For this review, take the finished solid that the model builds, in its own axes (mm). Face numbers are marked on the shaded views. A direction names the side the tool comes from. Round coordinates to 2 decimals unless told otherwise and drop trailing zeros. Order: outer loops, then holes, each group sorted by start corner. A loop starts at its lowest first (then second) coordinate and runs counter-clockwise, first axis right, second up. Notation, with made-up numbers: M -35.75,36.25 L -15.75,36.25 A18 ccw -15.75,46.25 Z; hole C -14,15.5 d2. An arc over 180 degrees is marked long. Write item = value, one per line. Start each with the question number.
from build123d import *

# Parameters (mm, degrees)
SKETCH5_W                 = 82
SKETCH5_H                 = 82
BOSS_EXTRUDE3_DEPTH       = 2
SKETCH9_W                 = 82
SKETCH9_H                 = 82
SKETCH9_W_2               = 75
SKETCH9_H_2               = 75
BOSS_EXTRUDE5_DEPTH       = 5
BOSS_EXTRUDE4_DEPTH       = 17.4
SKETCH7_W                 = 24
SKETCH7_H                 = 41
SKETCH7_W_2               = 27
SKETCH7_H_2               = 6
SKETCH7_W_3               = 53
CUT_EXTRUDE1_DEPTH        = 2
SKETCH10_W                = 6.5
SKETCH10_H                = 1.5
BOSS_EXTRUDE6_DEPTH       = 15
BOSS_EXTRUDE7_OUTLINE_W   = 82
BOSS_EXTRUDE7_OUTLINE_H   = 82
BOSS_EXTRUDE7_OUTLINE_W_2 = 80
BOSS_EXTRUDE7_OUTLINE_H_2 = 80
BOSS_EXTRUDE7_OUTLINE_W_3 = 77
BOSS_EXTRUDE7_OUTLINE_H_3 = 77
BOSS_EXTRUDE7_OUTLINE_W_4 = 75
BOSS_EXTRUDE7_OUTLINE_H_4 = 75
BOSS_EXTRUDE7_DEPTH       = 5
SKETCH12_W                = 28
SKETCH12_H                = 45
SKETCH12_W_2              = 24
SKETCH12_H_2              = 41
BOSS_EXTRUDE8_DEPTH       = 11.4


# Read off the part's stored shape, not the designer's step: Boss-Extrude7
with BuildPart() as part:
    # Sketch5 → Boss-Extrude3 (new body)
    with BuildSketch(Plane(origin=(0, 0, 0), x_dir=(1, 0, 0), z_dir=(0, 1, 0))):
        with Locations((40, 40)):
            Rectangle(SKETCH5_W, SKETCH5_H)
    extrude(amount=BOSS_EXTRUDE3_DEPTH)

    # Sketch9 → Boss-Extrude5 (add)
    with BuildSketch(Plane.XZ):
        with Locations((40, -40)):
            Rectangle(SKETCH9_W, SKETCH9_H)
        with Locations((40, -40)):
            Rectangle(SKETCH9_W_2, SKETCH9_H_2, mode=Mode.SUBTRACT)
    extrude(amount=BOSS_EXTRUDE5_DEPTH)

    # Sketch6 → Boss-Extrude4 (add)
    with BuildSketch(Plane.XZ):
        Polygon((35.5, -12.5), (35.5, -67.5), (73.5, -67.5), (73.5, -12.5), (57.5, -12.5), (57.5, -14.5), (71.5, -14.5), (71.5, -65.5), (37.5, -65.5), (37.5, -14.5), (51.5, -14.5), (51.5, -12.5), align=None)
    extrude(amount=BOSS_EXTRUDE4_DEPTH)

    # Sketch7 → Cut-Extrude1 (cut)
    with BuildSketch(Plane.XZ):
        with Locations((54.5, -40)):
            Rectangle(SKETCH7_W, SKETCH7_H)
        with Locations((64, -6.5)):
            Rectangle(SKETCH7_W_2, SKETCH7_H_2)
        with Locations((51, -73.5)):
            Rectangle(SKETCH7_W_3, SKETCH7_H_2)
    extrude(amount=-CUT_EXTRUDE1_DEPTH, mode=Mode.SUBTRACT)

    # Sketch10 → Boss-Extrude6 (add)
    with BuildSketch(Plane.XZ.offset(5)):
        with Locations((25.15, -0.75)):
            Rectangle(SKETCH10_W, SKETCH10_H)
    extrude(amount=BOSS_EXTRUDE6_DEPTH)

    # Boss-Extrude7 outline → Boss-Extrude7 (add)
    # profile 1 of 2: a face of its own
    with BuildSketch(Plane(origin=(0, -5, 0), x_dir=(-1, 0, 0), z_dir=(0, -1, 0))):
        with Locations((-40, 40)):
            Rectangle(BOSS_EXTRUDE7_OUTLINE_W, BOSS_EXTRUDE7_OUTLINE_H)
        with Locations((-40, 40)):
            Rectangle(BOSS_EXTRUDE7_OUTLINE_W_2, BOSS_EXTRUDE7_OUTLINE_H_2, mode=Mode.SUBTRACT)
    # profile 2 of 2: a face of its own
    with BuildSketch(Plane(origin=(0, -5, 0), x_dir=(-1, 0, 0), z_dir=(0, -1, 0))):
        with Locations((-40, 40)):
            Rectangle(BOSS_EXTRUDE7_OUTLINE_W_3, BOSS_EXTRUDE7_OUTLINE_H_3)
        with Locations((-40, 40)):
            Rectangle(BOSS_EXTRUDE7_OUTLINE_W_4, BOSS_EXTRUDE7_OUTLINE_H_4, mode=Mode.SUBTRACT)
    extrude(amount=BOSS_EXTRUDE7_DEPTH)

    # Sketch12 → Boss-Extrude8 (add)
    with BuildSketch(Plane.XZ):
        with Locations((54.5, -40)):
            Rectangle(SKETCH12_W, SKETCH12_H)
        with Locations((54.5, -40)):
            Rectangle(SKETCH12_W_2, SKETCH12_H_2, mode=Mode.SUBTRACT)
    extrude(amount=BOSS_EXTRUDE8_DEPTH)


solid = part.part
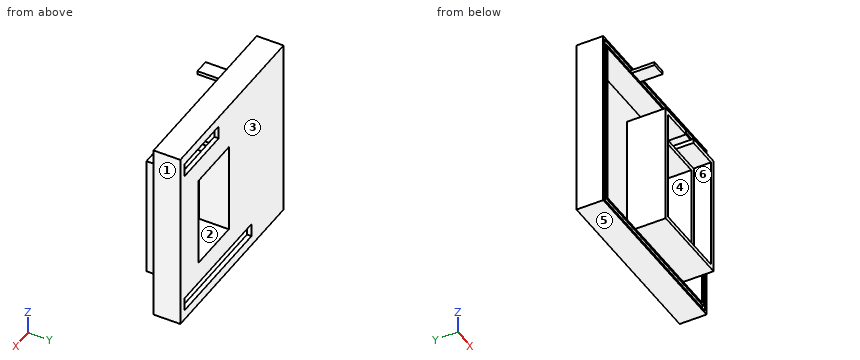
(1) We need section B-B, the plane y = -4. Write out the cut boundary in (x, z).
(2) We need section C-C, the plane y = -14.75. Write out the cut boundary in (x, z).
(3) For the marked faces 4, 5 and 6, list the 3-axis set-ups (+Z, -Z, +X, -X, +Y, -Y) from which the entire face can be reached by the end or side of a thin tool; tool diameter is ignored.
(4) For line 1 along Z through (x, y) = (55, -3.25); line 2 along Z through (x, y) = (26.5, -7.25); line 3 along X through (y, z) = (-4.5, -44), list the stretches that pass through material, from the lowest coordinate up.
(5) Draft analysis for pull direction X (two halves, no side actions). For the marked faces 1, 2 and 3, state which applies: released by +X, released by -X, zero draft, split by the parting line, or undercut.
(6) Insertion check: pin 1 (2 mm diameter, centred on x = 24, y = -16, fed in from -Z); pin 2 (5 mm diameter, centred on y = -13.5, z = -28.5, fed in from +X); pin 3 (1.2 mm diameter, centred on y = -13, z = -1, fed in from +X). Each pin has a flat end and moves straight along its axis. Give the tip position at first contact, or say it passes through.
(7) We need section D-D, the plane x = 12. Write out the cut boundary in (y, z).
Values:
q1.outline = M -1,-81 L 81,-81 L 81,1 L -1,1 Z; M 35.5,-67.5 L 73.5,-67.5 L 73.5,-12.5 L 57.5,-12.5 L 57.5,-14.5 L 71.5,-14.5 L 71.5,-65.5 L 37.5,-65.5 L 37.5,-14.5 L 51.5,-14.5 L 51.5,-12.5 L 35.5,-12.5 Z; M 40.5,-62.5 L 68.5,-62.5 L 68.5,-17.5 L 40.5,-17.5 Z; hole M 2.5,-77.5 L 77.5,-77.5 L 77.5,-2.5 L 2.5,-2.5 Z; hole M 42.5,-60.5 L 66.5,-60.5 L 66.5,-19.5 L 42.5,-19.5 Z
q2.outline = M 21.9,-1.5 L 28.4,-1.5 L 28.4,0 L 21.9,0 Z; M 35.5,-67.5 L 73.5,-67.5 L 73.5,-12.5 L 57.5,-12.5 L 57.5,-14.5 L 71.5,-14.5 L 71.5,-65.5 L 37.5,-65.5 L 37.5,-14.5 L 51.5,-14.5 L 51.5,-12.5 L 35.5,-12.5 Z
q3.face_4 = +Y, -Y
q3.face_5 = -Z, +X, -X, +Y, -Y
q3.face_6 = -Y
q4.line_1 = -81 to -77.5, -67.5 to -65.5, -62.5 to -60.5, -19.5 to -17.5, -2.5 to 1
q4.line_2 = -81 to -80, -78.5 to -77.5, -2.5 to 1
q4.line_3 = -1 to 2.5, 35.5 to 37.5, 40.5 to 42.5, 66.5 to 68.5, 71.5 to 73.5, 77.5 to 81
q5.face_1 = released by +X
q5.face_2 = undercut
q5.face_3 = zero draft
q6.pin_1 = -1.5
q6.pin_2 = 73.5
q6.pin_3 = 28.4
q7.outline = M -10,-81 L 2,-81 L 2,1 L -10,1 L -10,0 L -5,0 L -5,-1.5 L -10,-1.5 L -10,-2.5 L 0,-2.5 L 0,-77.5 L -10,-77.5 L -10,-78.5 L -5,-78.5 L -5,-80 L -10,-80 Z
